from build123d import *

# Parameters (mm, degrees)
F1_DEPTH = 18
F2_R     = 5


with BuildPart() as f1:
    # F0 (on Front) → F1 (new body)
    with BuildSketch(Plane.XZ):
        with BuildLine():
            ThreePointArc((12.0933866224, -14), (13.9727608958, -12.1248485743), (15.5643824163, -10))
            Line((15.5643824163, -10), (-15.5643824163, -10))
            ThreePointArc((-15.5643824163, -10), (-13.9727608958, -12.1248485743), (-12.0933866224, -14))
            Line((-12.0933866224, -14), (12.0933866224, -14))
        make_face()
        with BuildLine():
            Line((25, 8), (16.6808273176, 8))
            ThreePointArc((16.6808273176, 8), (17.7210793132, 5.311623855), (18.3310810811, 2.4942867515))
            ThreePointArc((18.3310810811, 2.4942867515), (20.2070006887, 1.8265127015), (21, 0))
            ThreePointArc((21, 0), (20.2070006887, -1.8265127015), (18.3310810811, -2.4942867515))
            ThreePointArc((18.3310810811, -2.4942867515), (17.358270198, -6.3984729219), (15.5643824163, -10))
            Line((15.5643824163, -10), (25, -10))
            Line((25, -10), (25, 8))
        make_face()
        with BuildLine():
            Line((2, 22), (2, 18.3915741577))
            ThreePointArc((2, 18.3915741577), (6.1642723241, 17.4428136123), (10, 15.5643824163))
            Line((10, 15.5643824163), (10, 22))
            Line((10, 22), (2, 22))
        make_face()
        with BuildLine():
            ThreePointArc((-10, 15.5643824163), (-6.1642723241, 17.4428136123), (-2, 18.3915741577))
            Line((-2, 18.3915741577), (-2, 22))
            Line((-2, 22), (-10, 22))
            Line((-10, 22), (-10, 15.5643824163))
        make_face()
        with BuildLine():
            ThreePointArc((-18.3310810811, 2.4942867515), (-17.7210793132, 5.311623855), (-16.6808273176, 8))
            Line((-16.6808273176, 8), (-25, 8))
            Line((-25, 8), (-25, -10))
            Line((-25, -10), (-15.5643824163, -10))
            ThreePointArc((-15.5643824163, -10), (-17.358270198, -6.3984729219), (-18.3310810811, -2.4942867515))
            ThreePointArc((-18.3310810811, -2.4942867515), (-21, 0), (-18.3310810811, 2.4942867515))
        make_face()
        with BuildLine():
            ThreePointArc((2, 9.2870878105), (3.6194093636, 8.7835002054), (5.123475383, 8))
            Line((5.123475383, 8), (10, 8))
            Line((10, 8), (10, 15.5643824163))
            ThreePointArc((10, 15.5643824163), (6.1642723241, 17.4428136123), (2, 18.3915741577))
            Line((2, 18.3915741577), (2, 9.2870878105))
        make_face()
        with BuildLine():
            Line((-10, 8), (-5.123475383, 8))
            ThreePointArc((-5.123475383, 8), (-3.6194093636, 8.7835002054), (-2, 9.2870878105))
            Line((-2, 9.2870878105), (-2, 18.3915741577))
            ThreePointArc((-2, 18.3915741577), (-6.1642723241, 17.4428136123), (-10, 15.5643824163))
            Line((-10, 15.5643824163), (-10, 8))
        make_face()
        with BuildLine():
            Line((10, 0), (9.5, 0))
            ThreePointArc((9.5, 0), (0, -9.5), (-9.5, 0))
            Line((-9.5, 0), (-10, 0))
            Line((-10, 0), (-10, 8))
            Line((-10, 8), (-16.6808273176, 8))
            ThreePointArc((-16.6808273176, 8), (-17.7210793132, 5.311623855), (-18.3310810811, 2.4942867515))
            ThreePointArc((-18.3310810811, 2.4942867515), (-16.6734872985, 1.7070006887), (-16, 0))
            ThreePointArc((-16, 0), (-16.6734872985, -1.7070006887), (-18.3310810811, -2.4942867515))
            ThreePointArc((-18.3310810811, -2.4942867515), (-17.358270198, -6.3984729219), (-15.5643824163, -10))
            Line((-15.5643824163, -10), (15.5643824163, -10))
            ThreePointArc((15.5643824163, -10), (17.358270198, -6.3984729219), (18.3310810811, -2.4942867515))
            ThreePointArc((18.3310810811, -2.4942867515), (16, 0), (18.3310810811, 2.4942867515))
            ThreePointArc((18.3310810811, 2.4942867515), (17.7210793132, 5.311623855), (16.6808273176, 8))
            Line((16.6808273176, 8), (10, 8))
            Line((10, 8), (10, 0))
        make_face()
        with BuildLine():
            Line((-10, 0), (-9.5, 0))
            ThreePointArc((-9.5, 0), (-8.3343570879, 4.5594398703), (-5.123475383, 8))
            Line((-5.123475383, 8), (-10, 8))
            Line((-10, 8), (-10, 0))
        make_face()
        with BuildLine():
            ThreePointArc((5.123475383, 8), (8.3343570879, 4.5594398703), (9.5, 0))
            Line((9.5, 0), (10, 0))
            Line((10, 0), (10, 8))
            Line((10, 8), (5.123475383, 8))
        make_face()
    extrude(amount=F1_DEPTH)

    # F2
    f2_edges = [f1.edges().sort_by_distance(p)[0] for p in [
        (-25, -9, 8),
        (-25, -9, -10),
        (25, -9, -10),
        (25, -9, 8),
        (10, -9, 8),
        (-10, -9, 8),
        (-12.093387, -9, -14),
        (12.093387, -9, -14),
    ]]
    fillet(f2_edges, radius=F2_R)


solid = f1.part
For this review, take the finished solid that the model builds, in its own axes (mm). A direction names the side the tool comes from. Round coordinates to 2 decimals unless told otherwise and drop trailing zeros. Order: outer loops, then holes, each group sorted by start corner. A loop starts at its lowest first (then second) coordinate and runs counter-clockwise, first axis right, second up. Notation, with made-up numbers: M -39,-6 L 15,-6 A14 ccw 15,4 Z; hole C -14,-4 d3. An arc over 180 degrees is marked long. Write each question's results on one line, items separated by ' | '. Start each with the question number.
1. Add section A-A (z = 16). State the section outline as (x, y) points, then the cut area to 3 significant figures.
2. Add section B-B (y = -6). State the section outline as (x, z) points.
3. Add section D-D (z = -11). State the section outline as (x, y) points, then the cut area to 3 significant figures.
4. To check wall thickness, follow L1, parallel to X at y = -5, z = 1; L2, parallel to X at y = -2, z = 15; L3, parallel to X at y = -5.75, z = 2. State the ranges of each line that lie inside material, in increasing order. Write a range as [from, to].
5. Clearance check with flat-ended pins moving along their axes: pin 1 Ø10 at (y, z) = (-6, 17.5) entering from -X; pin 2 Ø5.5 at (x, y) = (17, -8) entering from +Z; pin 3 Ø3.5 at (x, y) = (18.5, -9) entering from -Z. State where each tip first meets the part, or that it passes through.
6. Tool access review of faces 1 (the face through (-17, -9, 8)), 2 (the face through (0, -9, -14)), 3 (the face through (2, -9, 16)), 4 (the face through (18, -9, -10)): name each direction out of +Z, -Z, +X, -X, +Y, -Y from which nothing blocks a thin tool from reaching the whole face with its end or side.
7. Add section C-C (x = 0). State the section outline as (y, z) points, then the cut area to 3 significant figures.
Output values:
1) outline: M -10,-18 L -2,-18 L -2,0 L -10,0 Z; M 2,-18 L 10,-18 L 10,0 L 2,0 Z | area: 288 mm^2
2) outline: M -25,-5 A5 ccw -20,-10 L -15.56,-10 A18.5 ccw -13.79,-12.33 A5 ccw -10.06,-14 L 10.06,-14 A5 ccw 13.79,-12.33 A18.5 ccw 15.56,-10 L 20,-10 A5 ccw 25,-5 L 25,3 A5 ccw 20,8 L 15,8 A5 cw 10,13 L 10,22 L 2,22 L 2,9.29 A9.5 cw long -2,9.29 L -2,22 L -10,22 L -10,13 A5 cw -15,8 L -20,8 A5 ccw -25,3 Z; hole C -18.5,0 d5; hole C 18.5,0 d5
3) outline: M -14.87,-18 L 14.87,-18 L 14.87,0 L -14.87,0 Z | area: 535 mm^2
4) L1: [-25, -20.79], [-16.21, -9.45], [9.45, 16.21], [20.79, 25] | L2: [-10, -2], [2, 10] | L3: [-25, -20], [-17, -9.29], [9.29, 17], [20, 25]
5) pin 1: x = -10.03 | pin 2: z = 8.06 | pin 3: z = -10
6) face 1: +Z, -X, +Y, -Y | face 2: -Z, +X, -X, +Y, -Y | face 3: +Z, +Y, -Y | face 4: -Z, +X, +Y, -Y
7) outline: M -18,-14 L 0,-14 L 0,-9.5 L -18,-9.5 Z | area: 81.0 mm^2
